Autodesk Inventor part; units mm, degrees
ref_plane "YZ Plane" through (0, 0, 0) normal (1, 0, 0) x (0, 1, 0)
ref_plane "XZ Plane" through (0, 0, 0) normal (0, 1, 0) x (-1, 0, 0)
ref_plane "XY Plane" through (0, 0, 0) normal (0, 0, 1) x (1, 0, 0)
sketch "Sketch1" plane through (0, 0, 0) normal (1, 0, 0) x (0, 1, 0)
  line L0 (-1.5, 6.858) -> (1.5, 6.858)
  line L1 (1.5, 6.858) -> (1.5, -6.858)
  line L2 (1.5, -6.858) -> (-1.5, -6.858)
  line L3 (-1.5, -6.858) -> (-1.5, 6.858)
  line L4 (-1.5, 6.858) -> (1.5, -6.858) construction
  line L5 (1.5, 6.858) -> (-1.5, -6.858) construction
  line L6 (1.5, 6.858) -> (39.5, 6.858)
  line L7 (39.5, 6.858) -> (39.5, 9.858)
  line L8 (39.5, 9.858) -> (1.5, 9.858)
  line L9 (1.5, 9.858) -> (1.5, 6.858)
  line L10 (1.5, -6.858) -> (39.5, -6.858)
  line L11 (39.5, -6.858) -> (39.5, -9.858)
  line L12 (39.5, -9.858) -> (1.5, -9.858)
  line L13 (1.5, -9.858) -> (1.5, -6.858)
  line L14 (9.5, 6.858) -> (1.5, 6.858)
  line L15 (1.5, 6.858) -> (1.5, -0.142)
  line L16 (1.5, -0.142) -> (9.5, -0.142)
  line L17 (9.5, -0.142) -> (9.5, 6.858)
  line L18 (9.5, -6.858) -> (1.5, -6.858)
  line L19 (1.5, -6.858) -> (1.5, -0.142)
  line L20 (1.5, -0.142) -> (9.5, -0.142)
  line L21 (9.5, -0.142) -> (9.5, -6.858)
  line L22 (9.5, -0.142) -> (1.5, -0.142)
  line L23 (1.5, 6.858) -> (-1.5, 6.858)
  line L24 (-1.5, 6.858) -> (-1.5, 9.858)
  line L25 (-1.5, 9.858) -> (1.5, 9.858)
  line L26 (1.5, 9.858) -> (1.5, 6.858)
  line L27 (1.5, -6.858) -> (-1.5, -6.858)
  line L28 (-1.5, -6.858) -> (-1.5, -9.858)
  line L29 (-1.5, -9.858) -> (1.5, -9.858)
  line L30 (1.5, -9.858) -> (1.5, -6.858)
  point P0 (0, 0)
  dimension "d0" = 3
  dimension "d2" = 13.716
  dimension "d3" = 3
  dimension "d4" = 3
  dimension "d5" = 38
  dimension "d6" = 38
  dimension "d7" = 0
  dimension "d8" = 8
  dimension "d9" = 8
  dimension "d12" = 7
  dimension "d13" = 6.716
extrude "Extrusion1" add sketch "Sketch1" along normal blind 45
sketch "Sketch2" plane through (0, -1.5, 9.858) normal (0, 0, 1) x (1, 0, 0)
  line L0 (5, 7) -> (8.9446, 7)
  arc A0 (5, 7) -> (5, 0) centre (5, 3.5) ccw
  line L1 (8.9446, 0) -> (5, 0)
  arc A1 (13.3822, 14.1239) -> (31.6178, 14.1239) centre (22.5, 3.5) ccw
  line L2 (13.3822, 14.1239) -> (13.3822, 15.7096)
  line L3 (13.6751, 16.4167) -> (15.15, 17.8916)
  arc A2 (13.6751, 16.4167) -> (13.3822, 15.7096) centre (14.3822, 15.7096) ccw
  arc A3 (16.15, 20.3916) -> (15.15, 19.3916) centre (16.15, 19.3916) ccw
  line L4 (15.15, 19.3916) -> (15.15, 17.8916)
  line L5 (28.85, 20.3916) -> (16.15, 20.3916)
  arc A4 (29.85, 19.3916) -> (28.85, 20.3916) centre (28.85, 19.3916) ccw
  line L6 (29.85, 17.8916) -> (29.85, 19.3916)
  line L7 (31.3249, 16.4167) -> (29.85, 17.8916)
  line L8 (31.6178, 15.7096) -> (31.6178, 14.1239)
  arc A5 (31.6178, 15.7096) -> (31.3249, 16.4167) centre (30.6178, 15.7096) ccw
  line L9 (40, 7) -> (36.0554, 7)
  arc A6 (40, 0) -> (40, 7) centre (40, 3.5) ccw
  line L10 (36.0554, 0) -> (40, 0)
  line L11 (40, 7) -> (36.0554, 7)
  arc A7 (40, 0) -> (40, 7) centre (40, 3.5) ccw
  line L12 (36.0554, 0) -> (40, 0)
  line L13 (8.9446, 0) -> (5, 0)
  line L14 (36.0554, 0) -> (40, 0)
  line L15 (0, 41) -> (0, 0)
  line L16 (0, 0) -> (45, 0)
  line L17 (45, 41) -> (45, 0)
  line L18 (0, 41) -> (45, 41)
  line L19 (5, 7) -> (8.9446, 7)
  arc A8 (5, 7) -> (5, 0) centre (5, 3.5) ccw
sketch "Sketch3" plane through (0, -1.5, 9.858) normal (0, 0, 1) x (1, 0, 0)
  line L0 (0, 0) -> (45, 0)
  line L1 (45, 41) -> (45, 0)
  point P0 (0, 41)
  point P1 (0, 1.5)
  point P2 (5, 3.5)
  point P3 (40, 3.5)
  dimension "d16" = 35
  dimension "d18" = 5
  dimension "d19" = 45
  dimension "d20" = 3.5
  dimension "d21" = 3.5
hole "Hole1" at (5, 2, 9.858) at (40, 2, 9.858) direction (0, 0, -1) diameter 4.2 end through all
extrude "Extrusion2" cut sketch "Sketch2" against normal blind 0.82 contours A1 L2 A2 L3 L4 A3 L5 A4 L6 L7 A5 L8 L16 | L16 A1
sketch "Sketch4" plane through (0, -1.5, 9.858) normal (0, 0, 1) x (1, 0, 0)
  arc A0 (36.0554, 0) -> (31.6178, 14.1239) centre (22.5, 3.5) ccw
  line L0 (36.0554, 0) -> (45, 0)
  arc A1 (13.3822, 14.1239) -> (8.9446, 0) centre (22.5, 3.5) ccw
  circle A2 centre (5, 3.5) radius 2.1
  circle A3 centre (40, 3.5) radius 2.1
  arc A4 (5, 7) -> (5, 0) centre (5, 3.5) ccw
  line L1 (5, 7) -> (8.9446, 7)
  line L2 (8.9446, 0) -> (5, 0)
  arc A5 (13.3822, 14.1239) -> (31.6178, 14.1239) centre (22.5, 3.5) ccw
  arc A6 (13.3822, 14.1239) -> (31.6178, 14.1239) centre (22.5, 3.5) ccw
  line L3 (40, 7) -> (36.0554, 7)
  arc A7 (40, 0) -> (40, 7) centre (40, 3.5) ccw
  line L4 (36.0554, 0) -> (40, 0)
  point P0 (0, 1.5)
extrude "Extrusion3" cut sketch "Sketch4" against normal blind 0.82
sketch "Sketch5" plane through (0, -1.5, -9.858) normal (0, 0, -1) x (-1, 0, 0)
  circle A0 centre (-5, 3.5) radius 2.1
  circle A1 centre (-40, 3.5) radius 2.1
  line L0 (-34.959, 3.5) -> (-37.4795, -0.8656)
  line L1 (-37.4795, -0.8656) -> (-42.5205, -0.8656)
  line L2 (-42.5205, -0.8656) -> (-45.041, 3.5)
  line L3 (-45.041, 3.5) -> (-42.5205, 7.8656)
  line L4 (-42.5205, 7.8656) -> (-37.4795, 7.8656)
  line L5 (-37.4795, 7.8656) -> (-34.959, 3.5)
  line L6 (0.041, 3.5) -> (-2.4795, -0.8656)
  line L7 (-2.4795, -0.8656) -> (-7.5205, -0.8656)
  line L8 (-7.5205, -0.8656) -> (-10.041, 3.5)
  line L9 (-10.041, 3.5) -> (-7.5205, 7.8656)
  line L10 (-7.5205, 7.8656) -> (-2.4795, 7.8656)
  line L11 (-2.4795, 7.8656) -> (0.041, 3.5)
  point P0 (0, 1.5)
  point P1 (-40, 3.5)
  point P2 (-5, 3.5)
  dimension "d33" = 8.7312
  dimension "d34" = 8.7312
extrude "Extrusion4" cut sketch "Sketch5" against normal blind 3.175
sketch "Sketch6" plane through (0, 9.5, 6.858) normal (0, 1, 0) x (1, 0, 0)
  line L0 (7.5, 1.82) -> (37.5, 1.82)
  line L1 (37.5, 9.82) -> (7.5, 9.82)
  line L2 (7.5, 1.82) -> (7.5, 9.82)
  line L3 (37.5, 1.82) -> (37.5, 9.82)
  line L4 (7, 10.32) -> (38, 10.32)
  line L5 (38, 10.32) -> (38, 1.32)
  line L6 (38, 1.32) -> (7, 1.32)
  line L7 (7, 1.32) -> (7, 10.32)
  line L8 (8, 10.32) -> (37, 10.32)
  line L9 (37, 10.32) -> (37, 1.32)
  line L10 (37, 1.32) -> (8, 1.32)
  line L11 (8, 1.32) -> (8, 10.32)
  line L12 (0, 0) -> (45, 0)
  line L13 (8, 1.32) -> (37, 1.32)
  line L14 (37, 1.32) -> (37, 0)
  line L15 (37, 0) -> (8, 0)
  line L16 (8, 0) -> (8, 1.32)
  point P0 (0, 6.858)
  dimension "d37" = 0.5
  dimension "d56" = 1
  dimension "d57" = 1
chamfer "Chamfer1" distance 1 angle 45 2 edges at (22.5, 39.5, -6.858) (22.5, 39.5, 6.858)
sketch "Sketch7" plane through (0, 9.5, -6.858) normal (0, 0, 1) x (1, 0, 0)
  line L0 (0, 29) -> (0, 0)
  line L1 (0, 0) -> (45, 0)
  line L2 (45, 29) -> (45, 0)
  circle A0 centre (22.5, 10) radius 4.318
  line L3 (22.5, 10) -> (22.5, 20)
  circle A1 centre (22.5, 20) radius 2.159
  line L4 (20.341, 20) -> (20.341, 6.2605)
  line L5 (24.659, 20) -> (24.659, 6.2605)
  point P0 (0, -9.5)
  dimension "d43" = 8.636
  dimension "d45" = 10
  dimension "d46" = 4.318
  dimension "d47" = 22.5
  dimension "d48" = 45
  dimension "d49" = 10
extrude "Extrusion6" cut sketch "Sketch7" against normal through all
sketch "Sketch8" plane through (0, 9.5, -6.858) normal (0, 0, 1) x (1, 0, 0)
  arc A0 (20.341, 13.7395) -> (24.659, 13.7395) centre (22.5, 10) ccw
  line L0 (20.341, 13.7395) -> (20.341, 20)
  arc A1 (24.659, 20) -> (20.341, 20) centre (22.5, 20) ccw
  line L1 (24.659, 20) -> (24.659, 13.7395)
  line L2 (45, 29) -> (45, 0)
  circle A2 centre (22.5, 20) radius 4.318
  line L3 (18.182, 20) -> (18.182, 10)
  line L4 (26.818, 10) -> (26.818, 20)
  point P0 (0, -9.5)
  dimension "d52" = 4.318
  dimension "d53" = 8.636
extrude "Extrusion7" cut sketch "Sketch8" against normal blind 2 contours L0 A2 L1 A0 | A0 L3 A2 L0 | A2 L1 A1 L0 | A0 L1 A2 L4 picked at (24.9024, 17.6839)
extrude "Extrusion8" cut sketch "Sketch6" against normal through all contours L11 L1 L9 L0 | L0 L9 L6 L11 | L6 L14 L12 L16 | L11 L4 L9 L1
equation "\"d2\" = StretcherDepth"
equation "\"d6\" = d5"
equation "\"d9\" = d8"
equation "\"d47\" = 0.5 * d48"
equation "\"d53\" = 2 * d52"
properties part number "MotorClipV2" material "ABS Plastic"
Design review of the part built by this model. Coordinates are the model's own, in mm. A direction names the side the tool comes from. Give positions to 0.01 mm unless a question says otherwise; leave off trailing zeros. Order: outer loops, then holes, each group sorted by start corner. A loop starts at its lowest first (then second) coordinate and runs counter-clockwise, first axis right, second up. Notation, with made-up numbers: (45.5, -26) -> (76.5, -26) arc R8 cw to (76.5, -17) -> close; hole circle Ø11 at (80.25, 25). An arc over 180 degrees is marked (long way). Write each question's results on one line, items separated by ' | '. Start each with the question number.
Q1. Add section B-B on x = 22.5. Give the boundary of the cut face in (y, z).
Q2. Add section C-C on y = 25. Give the boundary of the cut face in (x, z), and give its area (3 significant figures).
Q3. Mouldability with a two-part tool opening along Y and no side actions: class faces 1 (the flat face through (43.778, 4.188, -8.293)), 2 (the flat face through (22.185, 39.007, -7.365)), 3 (the flat face through (17, 24, -6.858)) as +Y half, -Y half, draft (parallel to the pull), parting line (faces both ways), or undercut.
Q4. Machinability: for faces 4 (the flat face through (4, 4.2, -6.683)), 5 (the flat face through (37, 4, 2)), 6 (the flat face through (40, 6.366, -8)), 7 (the cylindrical face through (1.5, 2.1, 9.5)), which of the approach directions +Z, -Z, +X, -X, +Y, -Y give a long, thin tool a straight path to every point of the face, cutting with its end or side? Answer none if there is none.
Q5. Add section A-A on z = 0.75. Give the boundary of the cut face in (x, y), and give its area (3 significant figures).
Q6. Add section D-D on x = 41. Give the boundary of the cut face in (y, z).
Q7. Wall thickness on L1, parallel to X at y = 2, z = -3.5; L2, parallel to Y at x = 40, z = 2.75; L3, parallel to X at y = 19.5, z = -9.5: over which ranges is each line inside the solid? List them lowest first. Write a range as from..to.
Q8. For pin 1 (2 mm diameter, centred on x = 38.5, z = 6.5, fed in from +Y); pin 2 (5 mm diameter, centred on x = 40, y = 2, fed in from -Z); pin 3 (2.5 mm diameter, centred on x = 40, z = -8.5, fed in from -Y), all flat-tipped, find the tip position at first contact; note any pin that passes through.
Found:
1) outline: (-1.5, -9.86) -> (15.18, -9.86) -> (15.18, -6.86) -> (9.5, -6.86) -> (9.5, -3.46) -> (-1.5, -3.46) -> close; (-1.5, 6.86) -> (38.5, 6.86) -> (39.5, 7.86) -> (39.5, 9.86) -> (18.89, 9.86) -> (18.89, 9.04) -> (-1.5, 9.04) -> close; (31.66, -9.86) -> (39.5, -9.86) -> (39.5, -7.86) -> (38.5, -6.86) -> (33.82, -6.86) -> (33.82, -8.86) -> (31.66, -8.86) -> close
2) outline: (0, -9.86) -> (20.34, -9.86) -> (20.34, -8.86) -> (18.18, -8.86) -> (18.18, -6.86) -> (0, -6.86) -> close; (0, 6.86) -> (45, 6.86) -> (45, 9.86) -> (0, 9.86) -> close; (24.66, -9.86) -> (45, -9.86) -> (45, -6.86) -> (26.82, -6.86) -> (26.82, -8.86) -> (24.66, -8.86) -> close | area: 248 mm2
3) face 1: undercut | face 2: +Y half | face 3: draft
4) face 4: -Z | face 5: +Y, -Y | face 6: -Z, -Y | face 7: +Z
5) outline: (0, -1.5) -> (8, -1.5) -> (8, 9.5) -> (0, 9.5) -> close; (37, -1.5) -> (45, -1.5) -> (45, 9.5) -> (37, 9.5) -> close; hole circle Ø4.2 at (5, 2); hole circle Ø4.2 at (40, 2) | area: 148 mm2
6) outline: (-1.5, -6.68) -> (0.15, -6.68) -> (0.15, 9.04) -> (-1.35, 9.04) -> (-1.35, 9.86) -> (-1.5, 9.86) -> close; (3.85, -6.68) -> (6.37, -6.68) -> (6.37, -9.86) -> (39.5, -9.86) -> (39.5, -7.86) -> (38.5, -6.86) -> (9.5, -6.86) -> (9.5, 6.86) -> (38.5, 6.86) -> (39.5, 7.86) -> (39.5, 9.86) -> (5.35, 9.86) -> (5.35, 9.04) -> (3.85, 9.04) -> close
7) L1: x = 0..2.9, 7.1..37.9, 42.1..45 | L2: y = -1.5..-0.1, 4.1..9.5 | L3: x = 0..18.18, 26.82..45
8) pin 1: stops at y = 39.14 | pin 2: stops at z = -6.68 | pin 3: stops at y = 6.37
